Verification items for the finished model (mm, model axes). A direction names the side the tool comes from. Give positions to 0.01 mm unless a question says otherwise; leave off trailing zeros. Order: outer loops, then holes, each group sorted by start corner. A loop starts at its lowest first (then second) coordinate and runs counter-clockwise, first axis right, second up. Notation, with made-up numbers: (12.25, 19) -> (38.25, 19) arc R9 cw to (38.25, 24) -> close; hole circle Ø3 at (-11.75, 55). An arc over 180 degrees is marked (long way). Return JSON: item names as keys, results as strings. Group by question number.
(1) Cross-section at C-C on y = -1. Enter the section's corners in (x, z), then the cut area to 3 significant figures.
(2) Cross-section at D-D on z = 5.25. Enter the section's corners in (x, y).
(3) Release check for a two-part mould opening along X. For faces 4 (the face through (0, 2.286, -1)), 5 (the face through (0, 0, 3.619)), 6 (the face through (2.338, 0.736, 5.639)), 7 (the face through (-3, 0, -4.762)) record: pulls with the +X half, pulls with the -X half, needs draft (parallel to the pull), parting line crosses it, or undercut.
(4) Tool access check on faces 1 (the face through (2.286, 0, -1)), 2 (the face through (-2, 2, 4.762)), 3 (the face through (0, -3.81, 0)). Record the directions out of +Z, -Z, +X, -X, +Y, -Y that give a thin tool (end or side, any length) a straight path to the whole face; none if there is none.
(5) Cross-section at B-B on x = 0. Enter the section's corners in (y, z), then the cut area to 3 significant figures.
(6) Cross-section at A-A on z = 1.5. Enter the section's corners in (x, y), then the cut area to 3 significant figures.
(7) Thickness scan on line 1 along Y through (x, z) = (-2, 0.75); line 2 along Z through (x, y) = (2, 2.75). Record the ranges inside material, lowest first.
from build123d import *

# Parameters (mm, degrees)
F0_W     = 7.62
F0_H     = 7.620002
F1_DEPTH = 4.7625
F2_R     = 2.4511
F3_DEPTH = 1.778
F4_W     = 4.572
F4_H     = 4.572002
F5_DEPTH = 8.382


with BuildPart() as f1:
    # F0 (on Top) → F1 (new body, symmetric)
    with BuildSketch(Plane.XY):
        Rectangle(F0_W, F0_H)
    extrude(amount=F1_DEPTH, both=True)

    # F2 (on face) → F3 (join)
    with BuildSketch(Plane.XY.offset(4.7625)):
        Circle(F2_R)
    extrude(amount=F3_DEPTH)

    # F4 (on face) → F5 (cut)
    with BuildSketch(Plane(origin=(0, 0, -4.7625), x_dir=(1, 0, 0), z_dir=(0, 0, -1))):
        Rectangle(F4_W, F4_H)
    extrude(amount=-F5_DEPTH, mode=Mode.SUBTRACT)


solid = f1.part
Verdict:
{
 "1": {"outline": "(-3.81, -4.76) -> (-2.29, -4.76) -> (-2.29, 3.62) -> (2.29, 3.62) -> (2.29, -4.76) -> (3.81, -4.76) -> (3.81, 4.76) -> (2.24, 4.76) -> (2.24, 6.54) -> (-2.24, 6.54) -> (-2.24, 4.76) -> (-3.81, 4.76) -> close", "area": "42.2 mm²"},
 "2": {"outline": "circle Ø4.9 at (0, 0)"},
 "3": {"face 4": "undercut", "face 5": "undercut", "face 6": "parting line crosses it", "face 7": "needs draft"},
 "4": {"face 1": "-Z", "face 2": "+Z", "face 3": "+Z, -Z, +X, -X, -Y"},
 "5": {"outline": "(-3.81, -4.76) -> (-2.29, -4.76) -> (-2.29, 3.62) -> (2.29, 3.62) -> (2.29, -4.76) -> (3.81, -4.76) -> (3.81, 4.76) -> (2.45, 4.76) -> (2.45, 6.54) -> (-2.45, 6.54) -> (-2.45, 4.76) -> (-3.81, 4.76) -> close", "area": "43.0 mm²"},
 "6": {"outline": "(-3.81, -3.81) -> (3.81, -3.81) -> (3.81, 3.81) -> (-3.81, 3.81) -> close; hole (-2.29, -2.29) -> (2.29, -2.29) -> (2.29, 2.29) -> (-2.29, 2.29) -> close", "area": "37.2 mm²"},
 "7": {"line 1": "-3.81 to -2.29, 2.29 to 3.81", "line 2": "-4.76 to 4.76"}
}
